from build123d import *

# Parameters (mm, degrees)
SKETCH1_W           = 22.1
SKETCH1_H           = 6.3
BOSS_EXTRUDE1_DEPTH = 0.6
CUT_EXTRUDE1_DEPTH  = 24.73
SKETCH4_R           = 0.575
CUT_EXTRUDE2_DEPTH  = 2.54


with BuildPart() as part:
    # Sketch1 → Boss-Extrude1 (new body)
    with BuildSketch(Plane(origin=(0, 0, 0), x_dir=(1, 0, 0), z_dir=(0, 1, 0))):
        with Locations((11.05, 3.15)):
            Rectangle(SKETCH1_W, SKETCH1_H)
    extrude(amount=BOSS_EXTRUDE1_DEPTH)

    # Sketch3 → Cut-Extrude1 (cut)
    with BuildSketch(Plane(origin=(22.1, 0, 0), x_dir=(0, 0, -1), z_dir=(1, 0, 0))):
        Polygon((0, 0.6), (0, 0), (1.584478717, 0.6), align=None)
    extrude(amount=-CUT_EXTRUDE1_DEPTH, mode=Mode.SUBTRACT)

    # Sketch4 → Cut-Extrude2 (cut)
    with BuildSketch(Plane(origin=(0, 0.6, 0), x_dir=(1, 0, 0), z_dir=(0, 1, 0))):
        with Locations(Location((10.85, 5.189909292, 0), (0, 0, 270))):
            Circle(SKETCH4_R)
    extrude(amount=-CUT_EXTRUDE2_DEPTH, mode=Mode.SUBTRACT)


solid = part.part
Input: part model. Units: mm. Frame: model coordinates. Give positions to 0.01 mm unless a question says otherwise; leave off trailing zeros. Write each loop counter-clockwise with the first axis right and the second up, starting at its lowest first coordinate (ties: lowest second). Pieces come first, ordered by that corner, then holes. Notation, with made-up numbers: (-15, 32) -> (30, 32) arc R9 ccw to (30, 38) -> close; hole circle Ø7 at (26, 65). An arc over 180 degrees is marked (long way). Use one line per item in the form item = value. Start each with the question number.
1) Pin query (flat end, axial travel): pin 1 (0.7 mm diameter, centred on x = 10.85, z = -5.19, fed in from -Y). Return the tip coordinate at first contact, or that it passes through.
2) Ray query, probe 1 along X at (y, z) = (0.5, -5); probe 2 along X at (y, z) = (0.45, -5.5); probe 3 along Y at (x, z) = (20.5, -1). Return the intervals inside material, ascending. Write a range as from..to.
3) Section query B-B on z = -5. Return the cut outline in (x, y).
4) Section query A-A on x = 10.85. Return the cut outline in (y, z).
5) Section query D-D on z = -1.25. Return the cut outline in (x, y).
6) Section query C-C on y = 0.4. Return the cut outline in (x, z) (3 decimals), then the cut area to 3 significant figures.
7) Draft query along X for faces 1 (the flat face through (11.205, 0.296, -0.781)), 2 (the cylindrical face through (11.24, 0.3, -5.61)). Return one class per face: pulls with the +X half, pulls with the -X half, needs draft (parallel to the pull), parting line crosses it, or undercut.
Outcome:
q1.pin_1 = through
q2.probe_1 = 0..10.31, 11.39..22.1
q2.probe_2 = 0..10.37, 11.33..22.1
q2.probe_3 = 0..0.38
q3.outline = (0, 0) -> (10.31, 0) -> (10.31, 0.6) -> (0, 0.6) -> close; (11.39, 0) -> (22.1, 0) -> (22.1, 0.6) -> (11.39, 0.6) -> close
q4.outline = (0, -6.3) -> (0.6, -6.3) -> (0.6, -5.76) -> (0, -5.76) -> close; (0, -4.61) -> (0.6, -4.61) -> (0.6, -1.58) -> (0, 0) -> close
q5.outline = (0, 0) -> (22.1, 0) -> (22.1, 0.47) -> (0, 0.47) -> close
q6.outline = (0, -6.3) -> (22.1, -6.3) -> (22.1, -1.056) -> (0, -1.056) -> close; hole circle Ø1.15 at (10.85, -5.19)
q6.area = 115 mm^2
q7.face_1 = needs draft
q7.face_2 = undercut
